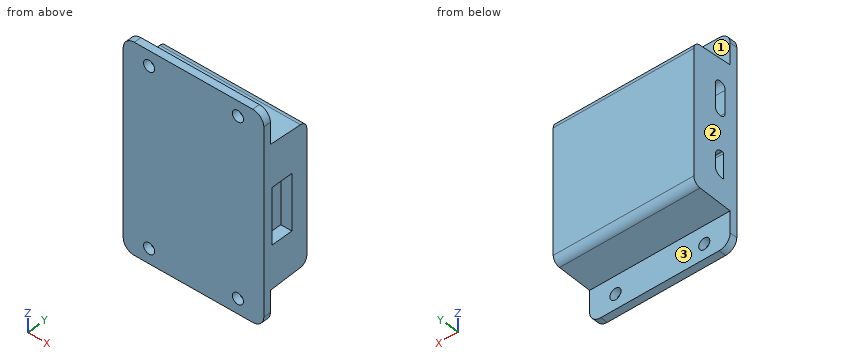
Autodesk Inventor part; units mm, degrees
ref_plane "YZ Plane" through (0, 0, 0) normal (1, 0, 0) x (0, 1, 0)
ref_plane "XZ Plane" through (0, 0, 0) normal (0, 1, 0) x (-1, 0, 0)
ref_plane "XY Plane" through (0, 0, 0) normal (0, 0, 1) x (1, 0, 0)
sketch "スケッチ1" plane through (0, 0, 0) normal (1, 0, 0) x (0, 1, 0)
  line L0 (-6.5, 27.75) -> (6.5, 27.75)
  line L1 (6.5, 27.75) -> (6.5, -27.75)
  line L2 (6.5, -27.75) -> (-6.5, -27.75)
  line L3 (-6.5, -27.75) -> (-6.5, 27.75)
  line L4 (-6.5, 27.75) -> (6.5, -27.75) construction
  line L5 (6.5, 27.75) -> (-6.5, -27.75) construction
  line L6 (6.5, 19) -> (-4.5, 19)
  line L7 (-4.5, 19) -> (-4.5, -19)
  line L8 (-4.5, -19) -> (6.5, -19)
  line L9 (6.5, -19) -> (6.5, 19)
  line L10 (-4.5, 27.75) -> (-4.5, 19)
  line L11 (-4.5, 19) -> (6.5, 18.5)
  line L12 (6.5, -18.5) -> (-4.5, -19)
  line L13 (-4.5, -19) -> (-4.5, -27.75)
  point P0 (0, 0)
  point P1 (6.5, 0)
  point P2 (6.5, 18.5)
  dimension "d0" = 13
  dimension "d1" = 55.5
  dimension "d2" = 11
  dimension "d3" = 38
  dimension "d4" = 0.5
  dimension "d5" = 0.5
extrude "押し出し1" add sketch "スケッチ1" along normal mid plane 38 contours L0 L10 L7 L13 L2 L3 | L11 L1 L12 L7
fillet "フィレット1" radius 2 2 edges at (0, 6.5, 18.5) (0, 6.5, -18.5)
sketch "スケッチ2" plane through (-19, -4.5, 27.75) normal (0, 1, 0) x (1, 0, 0)
  line L0 (7, 4) -> (31, 4) construction
  line L1 (7, 4) -> (31, 4) construction
  line L2 (0, 0) -> (38, 0) construction
  point P0 (19, 27.75)
  point P1 (19, 4)
  dimension "d9" = 24
  dimension "d10" = 0
  dimension "d11" = 4
hole "穴1" at (-12, -4.5, 23.75) at (12, -4.5, 23.75) direction (0, -1, 0) diameter 3 end through all
fillet "フィレット2" radius 3 2 edges at (19, -5.5, 27.75) (-19, -5.5, 27.75)
mirror "ミラー1" about plane through (0, 0, 0) normal (0, 0, 1) of "穴1", "フィレット2"
sketch "スケッチ3" plane through (19, 0, 0) normal (1, 0, 0) x (0, 0, -1)
  line L0 (-7.5, -4) -> (7.5, -4)
  line L1 (7.5, -4) -> (7.5, 2)
  line L2 (7.5, 2) -> (-7.5, 2)
  line L3 (-7.5, 2) -> (-7.5, -4)
  line L4 (-7.5, -4) -> (7.5, 2) construction
  line L5 (7.5, -4) -> (-7.5, 2) construction
  line L6 (-24.75, -6.5) -> (24.75, -6.5)
  point P0 (0, 0)
  point P1 (0, -1)
  dimension "d20" = 15
  dimension "d21" = 6
  dimension "d22" = 2.5
extrude "押し出し2" cut sketch "スケッチ3" against normal blind 3
sketch "スケッチ4" plane through (-19, 0, 0) normal (-1, 0, 0) x (0, 0, 1)
  line L0 (5.5, -1.5) -> (11.5, -1.5) construction
  line L1 (5.5, -3) -> (11.5, -3)
  line L2 (11.5, 0) -> (5.5, 0)
  arc A0 (5.5, 0) -> (5.5, -3) centre (5.5, -1.5) ccw
  arc A1 (11.5, -3) -> (11.5, 0) centre (11.5, -1.5) ccw
  line L3 (8.5, -1.5) -> (14.5, -1.5) construction
  line L4 (-12, -2.5) -> (-5, -2.5)
  line L5 (-5, -2.5) -> (-5, 0)
  line L6 (-5, 0) -> (-12, 0)
  line L7 (-12, 0) -> (-12, -2.5)
  line L8 (-12, -2.5) -> (-5, 0) construction
  line L9 (-5, -2.5) -> (-12, 0) construction
  point P0 (0, 0)
  point P1 (-8.5, -1.25)
  point P2 (-8.5, 0)
  point P3 (8.5, 0)
  dimension "d25" = 3
  dimension "d26" = 0
  dimension "d27" = 3
  dimension "d28" = 7
  dimension "d29" = 2.5
  dimension "d30" = 8.5
  dimension "d31" = 8.5
extrude "押し出し3" cut sketch "スケッチ4" against normal blind 5
fillet "フィレット3" radius 0.3 2 edges at (-16.5, -2.5, -12) (-16.5, -2.5, -5)
fillet "フィレット4" radius 2 2 edges at (-16.5, 0, -12) (-16.5, 0, -5)
equation "\"d5\" = d4"
properties part number "LiDAR_slave"
CAD build for the part. Positions are in the model's coordinates, mm. Face numbers are marked on the shaded views. A direction names the side the tool comes from. Coordinates: 2 decimals unless noted, no trailing zeros. Write each loop counter-clockwise with the first axis right and the second up, starting at its lowest first coordinate (ties: lowest second). Pieces come first, ordered by that corner, then holes.
(1) Cut at C-C, the plane x = -12. List the corners of the cut face in (y, z), and give its area (3 significant figures).
(2) 3-axis set-ups, long thin cutter, end or side, ignore diameter. For the marked faces 1, 2 and 3: which of +Z, -Z, +X, -X, +Y, -Y reach the whole face in a straight line?
(3) Cut at B-B, the plane z = 23.75. List the corners of the cut face in (x, y), and give its area (3 significant figures).
(4) Cut at A-A, the plane y = -5.25. List the corners of the cut face in (x, z), and give its area (3 significant figures).
(5) Drill centre lines: probe 1 along Z at (x, y) = (-12, -5.95); probe 2 along X at (y, z) = (-5.7, 23.75); probe 3 along Y at (x, z) = (-3, 21). Where is each one in solid material? Low to high.
(6) Flat gauge pins, fed straight in: pin 1 (2.5 mm diameter, centred on x = 12, z = -23.75, fed in from +Y); pin 2 (5 mm diameter, centred on x = -12.5, y = 1, fed in from +Z); pin 3 (5 mm diameter, centred on x = 13.5, y = 0.5, fed in from -Z); pin 4 (9.5 mm diameter, centred on x = 0, z = -25.5, fed in from +Y). Where does each tip first touch, or does it go through?
(7) Cut at D-D, the plane y = -1. List the corners of the cut face in (x, z).
Geometry says:
1. outline: (-6.5, -27.75) - (-4.5, -27.75) - (-4.5, -25.25) - (-6.5, -25.25) - close; (-6.5, -22.25) - (-4.5, -22.25) - (-4.5, -19) - (4.59, -18.59) arc R2 ccw to (6.5, -16.59) - (6.5, 16.59) arc R2 ccw to (4.59, 18.59) - (-4.5, 19) - (-4.5, 22.25) - (-6.5, 22.25) - close; (-6.5, 25.25) - (-4.5, 25.25) - (-4.5, 27.75) - (-6.5, 27.75) - close
1. area: 510 mm2
2. face 1: +Z, +X, -X, +Y
2. face 2: +Z, -Z, -X, +Y, -Y
2. face 3: -Z, +X, -X, +Y
3. outline: (-19, -6.5) - (-13.5, -6.5) - (-13.5, -4.5) - (-19, -4.5) - close; (-10.5, -6.5) - (10.5, -6.5) - (10.5, -4.5) - (-10.5, -4.5) - close; (13.5, -6.5) - (19, -6.5) - (19, -4.5) - (13.5, -4.5) - close
3. area: 64.0 mm2
4. outline: (-19, -24.75) arc R3 ccw to (-16, -27.75) - (16, -27.75) arc R3 ccw to (19, -24.75) - (19, 24.75) arc R3 ccw to (16, 27.75) - (-16, 27.75) arc R3 ccw to (-19, 24.75) - close; hole circle Ø3 at (-12, -23.75); hole circle Ø3 at (-12, 23.75); hole circle Ø3 at (12, -23.75); hole circle Ø3 at (12, 23.75)
4. area: 2,070 mm2
5. probe 1: z = -27.75 to -25.25, -22.25 to 22.25, 25.25 to 27.75
5. probe 2: x = -19 to -13.5, -10.5 to 10.5, 13.5 to 19
5. probe 3: y = -6.5 to -4.5
6. pin 1: passes through
6. pin 2: stops at z = 18.86
6. pin 3: stops at z = -18.89
6. pin 4: stops at y = -4.5
7. outline: (-19, -18.84) - (19, -18.84) - (19, -7.5) - (16, -7.5) - (16, 7.5) - (19, 7.5) - (19, 18.84) - (-19, 18.84) - (-19, 12.91) - (-14, 12.91) - (-14, 4.09) - (-19, 4.09) - (-19, -5.27) - (-14, -5.27) - (-14, -11.73) - (-19, -11.73) - close
